Source: CAD feature listing. Evaluate the final solid. Frame: model axes, mm. A direction names the side the tool comes from. Give positions to 0.01 mm unless a question says otherwise; leave off trailing zeros. Write each loop counter-clockwise with the first axis right and the second up, starting at its lowest first coordinate (ties: lowest second). Pieces come first, ordered by that corner, then holes. Notation, with made-up numbers: (87.25, -10) -> (102.25, -10) arc R16 ccw to (102.25, 11) -> close; hole circle Ø7 at (61, 30). An arc over 180 degrees is marked (long way). Write item = value, one per line.
Autodesk Inventor part; units mm, degrees
ref_plane "YZ Plane" through (0, 0, 0) normal (1, 0, 0) x (0, 1, 0)
ref_plane "XZ Plane" through (0, 0, 0) normal (0, 1, 0) x (-1, 0, 0)
ref_plane "XY Plane" through (0, 0, 0) normal (0, 0, 1) x (1, 0, 0)
sketch "Sketch1" plane through (0, 0, 0) normal (0, 0, 1) x (1, 0, 0)
  circle A0 centre (0, 0) radius 13.8
  circle A1 centre (0, 0) radius 11.5
  circle A2 centre (0, 0) radius 15.6
  circle A3 centre (0, 0) radius 12.5
  dimension "d0" = 27.6
  dimension "d1" = 23
  dimension "d2" = 31.2
  dimension "d3" = 25
extrude "Extrusion1" add sketch "Sketch1" along normal blind 1 contours A3
extrude "Extrusion2" add sketch "Sketch1" along normal blind 4 contours A0
sketch "Sketch2" plane through (0, 0, 4) normal (0, 0, 1) x (1, 0, 0)
  circle A0 centre (0, 0) radius 15.6
  circle A1 centre (0, 0) radius 12.5
extrude "Extrusion3" add sketch "Sketch2" along normal blind 1.5
extrude "Extrusion5" add sketch "Sketch2" against normal blind 1
sketch "Sketch3" plane through (0, 0, 5.5) normal (0, 0, 1) x (1, 0, 0)
  line L0 (0.5, 8.5) -> (-0.5, 8.5)
  line L1 (-0.5, 8.5) -> (-0.5, 16.5)
  line L2 (-0.5, 16.5) -> (0.5, 16.5)
  line L3 (0.5, 16.5) -> (0.5, 8.5)
  circle A0 centre (0, 0) radius 12.5
  line L4 (0.5, 8.5) -> (-0.5, 16.5) construction
  line L5 (-0.5, 8.5) -> (0.5, 16.5) construction
  point P0 (0, 12.5)
  dimension "d10" = 1
  dimension "d11" = 8
extrude "Extrusion4" cut sketch "Sketch3" against normal blind 10 contours L0 L1 A0 L3 | A0 L1 L2 L3 picked at (0.0556, 9.833)
properties part number "25mmFilterAdapter"
1) Draft query along X for faces 1 (the flat face through (-0.5, 13.5, 3.4)), 2 (the flat face through (-9.3, -7.1, 0)). Return one class per face: pulls with the +X half, pulls with the -X half, needs draft (parallel to the pull), parting line crosses it, or undercut.
Computed:
face_1 = undercut
face_2 = needs draft
2) Cut plane B-B (x = 0). Return the cut outline in (y, z).
Computed:
outline = (-15.6, 3) -> (-13.8, 3) -> (-13.8, 0) -> (-11.5, 0) -> (-11.5, 1) -> (-12.5, 1) -> (-12.5, 5.5) -> (-15.6, 5.5) -> close
3) Cut plane D-D (z = 3.5). Return the cut outline in (x, y).
Computed:
outline = (-0.5, 12.49) -> (-0.5, 15.59) arc R15.6 ccw (long way) to (0.5, 15.59) -> (0.5, 12.49) arc R12.5 cw (long way) to start
4) Material intervals for L1, parallel to X at y = 0, z = 2.55; L2, parallel to X at y = 0, z = 4.2; L3, parallel to Y at x = 8.5, z = 1.3, sorted ascending.
Computed:
L1 = -13.8 to -12.5, 12.5 to 13.8
L2 = -15.6 to -12.5, 12.5 to 15.6
L3 = -10.87 to -9.17, 9.17 to 10.87
5) Cut plane A-A (y = 3). Return the cut outline in (x, z).
Computed:
outline = (-15.31, 3) -> (-13.47, 3) -> (-13.47, 0) -> (-11.1, 0) -> (-11.1, 1) -> (-12.13, 1) -> (-12.13, 5.5) -> (-15.31, 5.5) -> close; (11.1, 0) -> (13.47, 0) -> (13.47, 3) -> (15.31, 3) -> (15.31, 5.5) -> (12.13, 5.5) -> (12.13, 1) -> (11.1, 1) -> close
6) Access query for faces 3 (the flat face through (-6, -10, 1)), 4 (the flat face through (0.5, 13.6, 3.4)), 5 (the flat face through (1, -14, 3)). Directions: +Z, -Z, +X, -X, +Y, -Y. A direction counts if a zero-diameter tool reaches every point of the face in a straight line with its end or side. Return the directions, or none.
Computed:
face_3 = +Z
face_4 = +Z, -Z, +Y
face_5 = -Z
7) Cut plane C-C (x = 11). Return the cut outline in (y, z), then the cut area to 3 significant figures.
Computed:
outline = (-11.06, 3) -> (-8.33, 3) -> (-8.33, 0) -> (-3.35, 0) -> (-3.35, 1) -> (-5.94, 1) -> (-5.94, 5.5) -> (-11.06, 5.5) -> close; (3.35, 0) -> (8.33, 0) -> (8.33, 3) -> (11.06, 3) -> (11.06, 5.5) -> (5.94, 5.5) -> (5.94, 1) -> (3.35, 1) -> close
area = 45.2 mm²
8) Contact query for flat-ended pins moving along their axis: pin 1 (3 mm diameter, centred on x = 12.5, z = 1, fed in from -Y); pin 2 (2 mm diameter, centred on y = 14.5, z = 2.5, fed in from -X); pin 3 (2 mm diameter, centred on x = -4, z = 3, fed in from +Y); pin 4 (10 mm diameter, centred on x = 4, y = 9, fed in from +Z). Output: stop coordinate, or through.
Computed:
pin_1 = -8.33
pin_2 = -7.58
pin_3 = 15.31
pin_4 = 5.5
